Drawing for the job (mm, zero at the part's lowest x, y, z). Coordinates: 2 decimals unless noted, no trailing zeros. Write each loop counter-clockwise with the first axis right and the second up, starting at its lowest first coordinate (ties: lowest second). Pieces come first, ordered by that corner, then holes. Notation, with made-up numbers: M 48,1 L 107,1 A14 cw 107,11 Z; hole C 84,62 d6. An arc over 180 degrees is marked long. Put each result on its own line as item: value. Start each with the question number.
Q1. Cut at C-C (x = 127). Write the cut outline in (y, z).
Q2. Drop flat-ended pins along their axis: pin 1 (1.5 mm diameter, centred on y = 2, z = 54.5, fed in from +X) (1 decimal); pin 2 (8 mm diameter, centred on x = 153.5, z = 76, fed in from +Y); pin 3 (1 mm diameter, centred on y = 5.5, z = 144, fed in from +X) (1 decimal); pin 4 (1 mm diameter, centred on y = 3, z = 41.5, fed in from +X). Give the stop position or say it passes through.
Q3. Cut at A-A (y = 4.75). Write the cut outline in (x, z) (1 decimal), then the cut area to 3 significant figures.
Q4. Drill centre lines: line 1 along Z through (x, y) = (44.5, 5.5) (1 decimal); line 2 along Z through (x, y) = (99, 3.5) (1 decimal); line 3 along Z through (x, y) = (67, 7) (1 decimal). Where is each one in solid material? Low to high.
Q5. Cut at B-B (z = 77). Write the cut outline in (x, y).
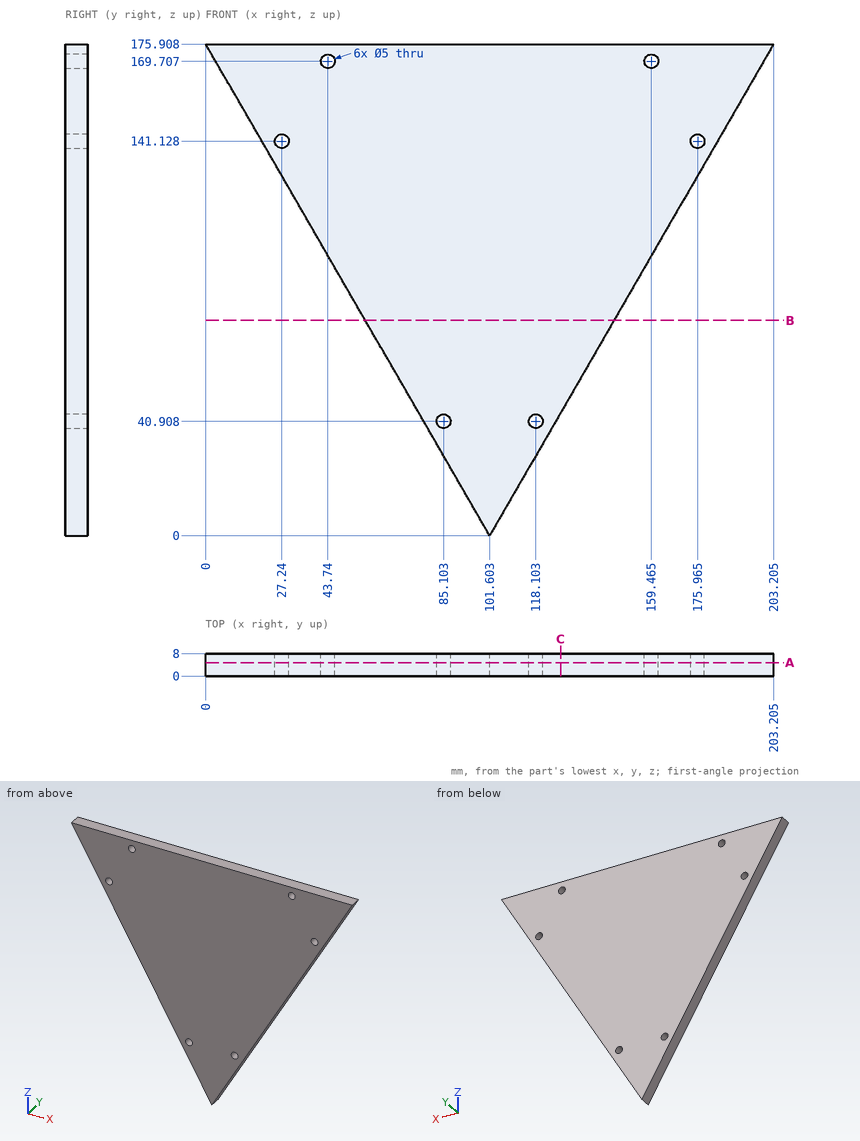
Computed values:
1. outline: M 0,43.97 L 8,43.97 L 8,175.91 L 0,175.91 Z
2. pin 1: x = 133.5
2. pin 2: through
2. pin 3: x = 185.1
2. pin 4: x = 125.86
3. outline: M 0,175.9 L 101.6,0 L 203.2,175.9 Z; hole C 27.2,141.1 d5; hole C 43.7,169.7 d5; hole C 85.1,40.9 d5; hole C 118.1,40.9 d5; hole C 159.5,169.7 d5; hole C 176,141.1 d5
3. area: 17,800 mm2
4. line 1: 98.9 to 167.3, 172.1 to 175.9
4. line 2: 4.5 to 175.9
4. line 3: 59.9 to 175.9
5. outline: M 57.13,0 L 146.08,0 L 146.08,8 L 57.13,8 Z
